Part print with two shaded views. Sizes in mm from the minimum x, y, z corner. Coordinates: 2 decimals unless noted, no trailing zeros. Loops run counter-clockwise (first coordinate to the right, second up) from the corner with the lowest first, then second, coordinate; pieces in that order, holes last. Notation, with made-up numbers: M -35.5,-8 L 14.5,-8 A11 ccw 14.5,11 Z; hole C 21,49.5 d1. An arc over 180 degrees is marked long. Use CSV: the item, a comma, the result in double quotes. Start each with the question number.
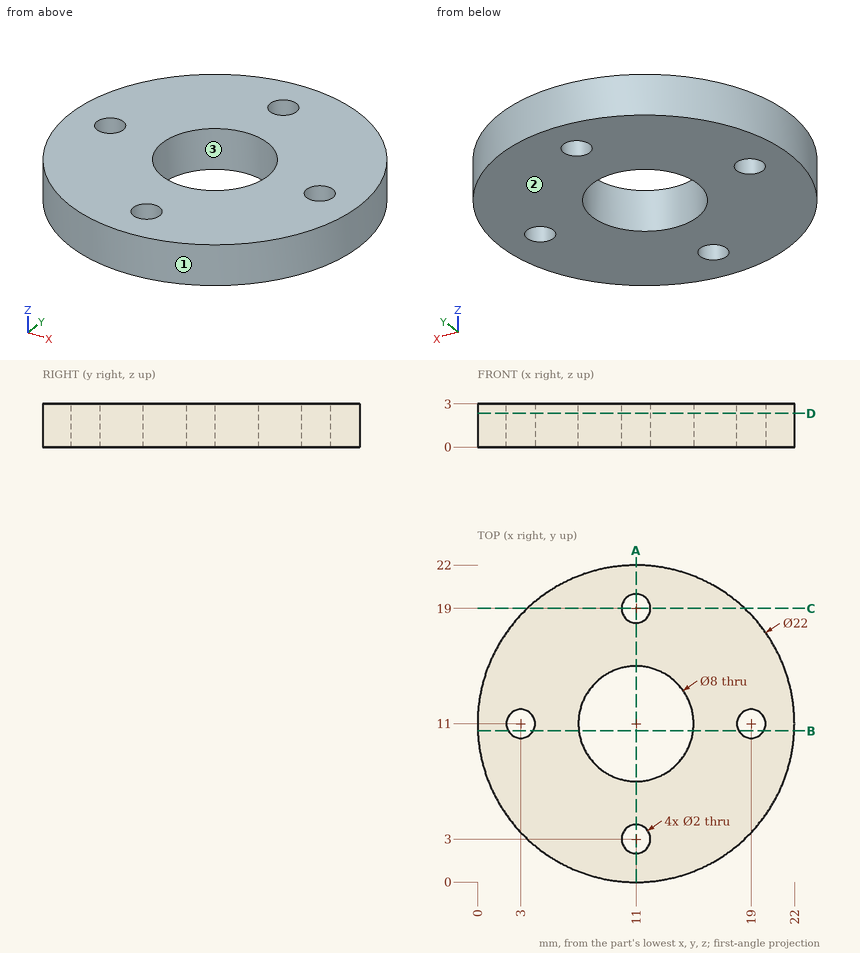
1. Slice it at C-C, the plane y = 19. List the corners of the cut face in (x, z), and give its area (3 significant figures).
2. Slice it at A-A, the plane x = 11. List the corners of the cut face in (y, z), and give its area (3 significant figures).
3. Pin check, flat tips, straight feed: pin 1 (2.5 mm diameter, centred on x = 3, y = 11, fed in from -Z); pin 2 (1.5 mm diameter, centred on y = 13, z = 2, fed in from -X). Stop position of each tip, or through.
4. Slice it at D-D, the plane z = 2.35. List the corners of the cut face in (x, y).
5. Wall check: probe 1 along Y at (x, z) = (11, 1.7); probe 2 along X at (y, z) = (19.75, 1.1); probe 3 along X at (y, z) = (18.75, 2). Give the ranges that are in metal, low to high.
6. Two-plate mould, pull along X, no slides. Class the marked faces 1, 2 and 3: pulls with the +X half, pulls with the -X half, needs draft (parallel to the pull), parting line crosses it, or undercut.
7. Slice it at B-B, the plane y = 10.5. List the corners of the cut face in (x, z), and give its area (3 significant figures).
Found:
1,outline,"M 3.45,0 L 10,0 L 10,3 L 3.45,3 Z; M 12,0 L 18.55,0 L 18.55,3 L 12,3 Z"
1,area,"39.3 mm^2"
2,outline,"M 0,0 L 2,0 L 2,3 L 0,3 Z; M 4,0 L 7,0 L 7,3 L 4,3 Z; M 15,0 L 18,0 L 18,3 L 15,3 Z; M 20,0 L 22,0 L 22,3 L 20,3 Z"
2,area,"30.0 mm^2"
3,pin 1,"z = 0"
3,pin 2,"x = 0.07"
4,outline,"C 11,11 d22; hole C 3,11 d2; hole C 11,11 d8; hole C 11,3 d2; hole C 11,19 d2; hole C 19,11 d2"
5,probe 1,"0 to 2, 4 to 7, 15 to 18, 20 to 22"
5,probe 2,"4.33 to 10.34, 11.66 to 17.67"
5,probe 3,"3.19 to 10.03, 11.97 to 18.81"
6,face 1,"parting line crosses it"
6,face 2,"needs draft"
6,face 3,"undercut"
7,outline,"M 0.01,0 L 2.13,0 L 2.13,3 L 0.01,3 Z; M 3.87,0 L 7.03,0 L 7.03,3 L 3.87,3 Z; M 14.97,0 L 18.13,0 L 18.13,3 L 14.97,3 Z; M 19.87,0 L 21.99,0 L 21.99,3 L 19.87,3 Z"
7,area,"31.7 mm^2"
